from build123d import *

# Parameters (mm, degrees)
F1_DEPTH  = 10
F1_FACE_W = 6.7
F1_FACE_H = 10
F2_DEPTH  = 0.5
F3_DEPTH  = 190


with BuildPart() as f1:
    # F0 (on Front) → F1 (new body)
    with BuildSketch(Plane.XZ):
        Polygon((-3.35, 4), (-8.35, 4), (-8.35, -4), (8.35, -4), (8.35, 4), (3.35, 4), (3.35, -2), (-3.35, -2), align=None)
    extrude(amount=F1_DEPTH)

    # F1_face (on face) → F2 (join)
    with BuildSketch(Plane(origin=(0, -5, -2), x_dir=(1, 0, 0), z_dir=(0, 0, 1))):
        Rectangle(F1_FACE_W, F1_FACE_H)
    extrude(amount=F2_DEPTH)

    # F2_face (on face) → F3 (join)
    with BuildSketch(Plane(origin=(0, -10, -0.476098), x_dir=(1, 0, 0), z_dir=(0, -1, 0))):
        Polygon((-3.35, 4.476098), (-8.35, 4.476098), (-8.35, -3.523902), (8.35, -3.523902), (8.35, 4.476098), (3.35, 4.476098), (3.35, -1.023902), (-3.35, -1.023902), align=None)
    extrude(amount=F3_DEPTH)


solid = f1.part
The listing builds one solid part. Answer for the finished solid, in the listing's coordinates (mm). A direction names the side the tool comes from. Give positions to 0.01 mm unless a question says otherwise; leave off trailing zeros. Write each loop counter-clockwise with the first axis right and the second up, starting at its lowest first coordinate (ties: lowest second). Pieces come first, ordered by that corner, then holes. Notation, with made-up numbers: (28, -37) - (33, -37) arc R11 cw to (33, -16) - close; hole circle Ø5 at (-39, 3). An arc over 180 degrees is marked (long way). One line per question, with ' | ' between items. Start each with the question number.
1. Straight lines are drawn through the part: line 1 (X direction, y = -47, z = 1); line 2 (Z direction, x = 0, y = -47). For each, find the intervals that lie inside material, in ascending order.
2. Section B-B, the plane y = -99 is taken. Determine the outline of the cut face in (x, z).
3. Determine the mould class of faces 3 (the face through (8.35, -99, 0)), 4 (the face through (0, -99, -4)), 5 (the face through (3.35, -99, 1)) for opening direction X: +X half, -X half, draft (parallel to the pull), parting line (faces both ways), or undercut.
4. Given P1, Ø3.5, axis at x = -1, y = -94, coming from the +Z side, flat-ended and moving along its own axis, determine where the tip first touches the part or whether it passes through.
5. For faces 1 (the face through (0, -99, -1.5)), 2 (the face through (-8.35, -99, 0)), determine the directions among +Z, -Z, +X, -X, +Y, -Y from which every point of the face is accessible in a straight line to the end or side of a thin tool.
6. Section C-C, the plane x = 0 is taken. Determine the outline of the cut face in (y, z).
7. Section A-A, the plane z = 0.25 is taken. Determine the outline of the cut face in (x, y), then the cut area to 3 significant figures.
Result:
1) line 1: x = -8.35 to -3.35, 3.35 to 8.35 | line 2: z = -4 to -1.5
2) outline: (-8.35, -4) - (8.35, -4) - (8.35, 4) - (3.35, 4) - (3.35, -1.5) - (-3.35, -1.5) - (-3.35, 4) - (-8.35, 4) - close
3) face 3: +X half | face 4: draft | face 5: undercut
4) P1: stops at z = -1.5
5) face 1: +Z, +Y, -Y | face 2: +Z, -Z, -X, +Y, -Y
6) outline: (-200, -4) - (0, -4) - (0, -1.5) - (-200, -1.5) - close
7) outline: (-8.35, -200) - (-3.35, -200) - (-3.35, 0) - (-8.35, 0) - close; (3.35, -200) - (8.35, -200) - (8.35, 0) - (3.35, 0) - close | area: 2,000 mm2
